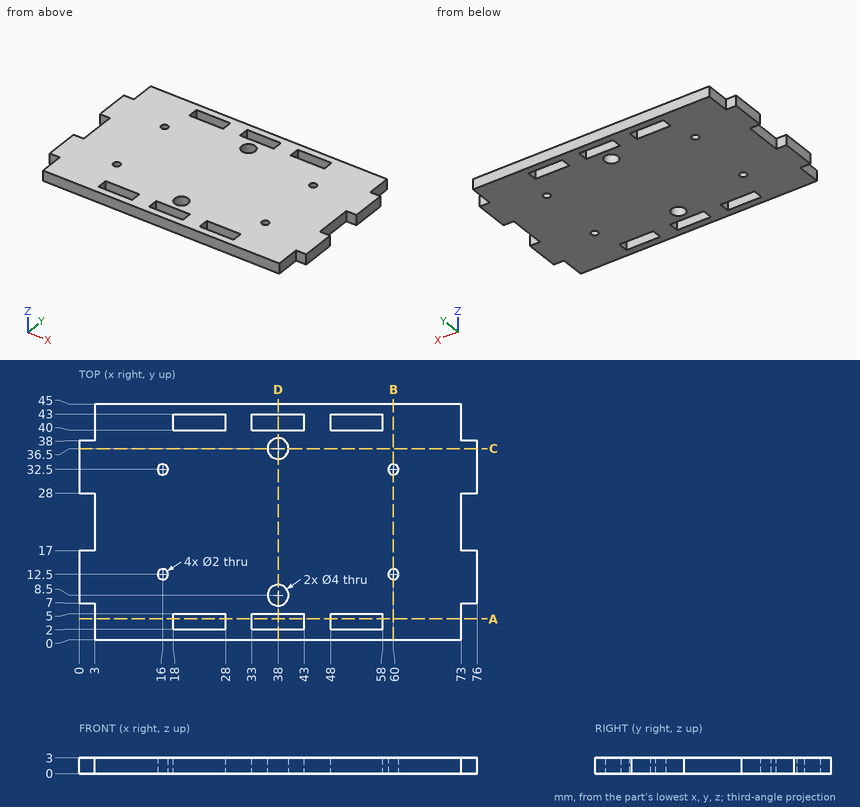
Job drawing, mm, ordinate dimensions from the low corner. One solid piece. Round coordinates to 2 decimals unless told otherwise and drop trailing zeros. Loops run counter-clockwise (first coordinate to the right, second up) from the corner with the lowest first, then second, coordinate; pieces in that order, holes last. Notation, with made-up numbers: M 38,7.5 L 83,7.5 A4 ccw 83,14.5 Z; hole C 4.25,-5 d1. An arc over 180 degrees is marked long. Answer as CSV lines item,"result".
1. Flat gauge pins, fed straight in: P1, Ø1.5, axis at y = 42, z = 1.5, coming from the +X side; P2, Ø0.9, axis at y = 24.5, z = 1, coming from the -X side. Where does each tip first touch, or does it go through?
Resolved:
P1,"stops at x = 73"
P2,"stops at x = 3"
2. Cut at B-B on x = 60. Write the cut outline in (y, z).
Resolved:
outline,"M 0,0 L 11.5,0 L 11.5,3 L 0,3 Z; M 13.5,0 L 31.5,0 L 31.5,3 L 13.5,3 Z; M 33.5,0 L 45,0 L 45,3 L 33.5,3 Z"
3. Wall check: probe 1 along X at (y, z) = (32.5, 1.95); probe 2 along Y at (x, z) = (54.5, 1.2); probe 3 along Y at (x, z) = (60, 1.65). Give the ranges that are in metal, low to high. Write a range as [from, to].
Resolved:
probe 1,"x = [0, 15], [17, 59], [61, 76]"
probe 2,"y = [0, 2], [5, 40], [43, 45]"
probe 3,"y = [0, 11.5], [13.5, 31.5], [33.5, 45]"
4. Cut at A-A on y = 4. Write the cut outline in (x, z).
Resolved:
outline,"M 3,0 L 18,0 L 18,3 L 3,3 Z; M 28,0 L 33,0 L 33,3 L 28,3 Z; M 43,0 L 48,0 L 48,3 L 43,3 Z; M 58,0 L 73,0 L 73,3 L 58,3 Z"
5. Cut at D-D on x = 38. Write the cut outline in (y, z), then the cut area to 3 significant figures.
Resolved:
outline,"M 0,0 L 2,0 L 2,3 L 0,3 Z; M 5,0 L 6.5,0 L 6.5,3 L 5,3 Z; M 10.5,0 L 34.5,0 L 34.5,3 L 10.5,3 Z; M 38.5,0 L 40,0 L 40,3 L 38.5,3 Z; M 43,0 L 45,0 L 45,3 L 43,3 Z"
area,"93.0 mm²"
6. Cut at C-C on y = 36.5. Write the cut outline in (x, z), then the cut area to 3 significant figures.
Resolved:
outline,"M 0,0 L 36,0 L 36,3 L 0,3 Z; M 40,0 L 76,0 L 76,3 L 40,3 Z"
area,"216 mm²"
